from build123d import *

# Parameters (mm, degrees)
F0_R     = 5
F0_R_2   = 4
F1_DEPTH = 8
F2_DEPTH = 12


with BuildPart() as f1:
    # F0 (on Top) → F1 (new body)
    with BuildSketch(Plane.XY):
        Circle(F0_R)
        Circle(F0_R_2, mode=Mode.SUBTRACT)
    extrude(amount=F1_DEPTH)

    # F0 (on Top) → F2 (join)
    with BuildSketch(Plane.XY):
        Circle(F0_R_2)
    extrude(amount=F2_DEPTH)

    # F3 (on Front) → F4 (revolve, cut)
    with BuildSketch(Plane.XZ):
        Polygon((2.1, -3.645375), (2.1, 0), (2.1, 7.9), (0, 10), (0, -3.645375), align=None)
    revolve(axis=Axis((0, 0, 3.177312), (0, 0, 1)), mode=Mode.SUBTRACT)


solid = f1.part
Source: CAD feature listing. Evaluate the final solid. Frame: model axes, mm. A direction names the side the tool comes from. Give positions to 0.01 mm unless a question says otherwise; leave off trailing zeros. Order: outer loops, then holes, each group sorted by start corner. A loop starts at its lowest first (then second) coordinate and runs counter-clockwise, first axis right, second up. Notation, with made-up numbers: (29.5, -16.5) -> (77.5, -16.5) arc R37 ccw to (77.5, 20.5) -> close; hole circle Ø7 at (48.25, -9.5). An arc over 180 degrees is marked (long way). Write item = value, one per line.
Q1. Set-up query: faces 4 (the face through (2.003, 0.631, 4.005)), 5 (the face through (-1.08, -4.88, 3.94)). Return all of +Z, -Z, +X, -X, +Y, -Y with unobstructed straight access to the full face (end or side cutting, diameter ignored); none if empty.
Data:
face_4 = -Z
face_5 = +Z, -Z
Q2. Material intervals for line 1 (Y direction, x = 0, z = 5.75); line 2 (Z direction, x = 2.75, y = 3.5); line 3 (X direction, y = 1.75, z = 3), sorted ascending. Write a range as from..to.
Data:
line_1 = -5..-2.1, 2.1..5
line_2 = 0..8
line_3 = -4.68..-1.16, 1.16..4.68
Q3. Cut plane A-A, the plane y = -2.75. Output: boundary loops of the cut face in (x, z).
Data:
outline = (-4.18, 0) -> (4.18, 0) -> (4.18, 8) -> (2.9, 8) -> (2.9, 12) -> (-2.9, 12) -> (-2.9, 8) -> (-4.18, 8) -> close
Q4. Cut plane B-B, the plane z = 6.75. Output: boundary loops of the cut face in (x, y), and give its area (3 significant figures).
Data:
outline = circle Ø10 at (0, 0); hole circle Ø4.2 at (0, 0)
area = 64.7 mm^2
Q5. Cut plane C-C, the plane z = 11. Output: boundary loops of the cut face in (x, y), and give its area (3 significant figures).
Data:
outline = circle Ø8 at (0, 0)
area = 50.3 mm^2
Q6. Pull-direction query (Y, two-part tool) for faces 1 (the face through (1, -2.2, 0)), 2 (the face through (-0.45, -0.35, 9.43)), 3 (the face through (-0.867, -3.905, 9.972)); classes: released by +Y, released by -Y, zero draft, split by the parting line, or undercut.
Data:
face_1 = zero draft
face_2 = undercut
face_3 = split by the parting line
Q7. Cut plane D-D, the plane y = 4.25. Output: boundary loops of the cut face in (x, z), and give its area (3 significant figures).
Data:
outline = (-2.63, 0) -> (2.63, 0) -> (2.63, 8) -> (-2.63, 8) -> close
area = 42.1 mm^2
Q8. Pin query (flat end, axial travel): pin 1 (1 mm diameter, centred on y = -2, z = 7, fed in from +X); pin 2 (1 mm diameter, centred on x = 0.5, z = 10.5, fed in from -Y). Return the tip coordinate at first contact, or that it passes through.
Data:
pin_1 = 4.77
pin_2 = -4
